```python
from build123d import *

# Parameters (mm, degrees)
F0_W      = 42
F0_H      = 17
F1_DEPTH  = 7
F4_DEPTH  = 25
F5_W      = 42
F5_H      = 5.6745335534
F6_DEPTH  = 10
F7_R      = 1.675
F8_DEPTH  = 25
F9_DEPTH  = 25
F10_W     = 5.7
F10_H     = 7
F11_DEPTH = 5
F12_DEPTH = 2


with BuildPart() as f1:
    # F0 (on Top) → F1 (new body)
    with BuildSketch(Plane.XY):
        with Locations((21, 8.5)):
            Rectangle(F0_W, F0_H)
    extrude(amount=F1_DEPTH)

    # F3 (on face) → F4 (cut)
    with BuildSketch(Plane(origin=(0, 17, 0), x_dir=(-1, 0, 0), z_dir=(0, 1, 0))):
        with BuildLine():
            ThreePointArc((-38.175, 3.5), (-36.5, 1.825), (-34.825, 3.5))
            ThreePointArc((-34.825, 3.5), (-36.5, 5.175), (-38.175, 3.5))
        make_face()
    extrude(amount=-F4_DEPTH, mode=Mode.SUBTRACT)

    # F5 (on face) → F6 (join)
    with BuildSketch(Plane.XY.offset(7)):
        with Locations((21, 14.1627332233)):
            Rectangle(F5_W, F5_H)
    extrude(amount=F6_DEPTH)

    # F7 (on face) → F8 (cut)
    with BuildSketch(Plane(origin=(0, 17, 0), x_dir=(-1, 0, 0), z_dir=(0, 1, 0))):
        with Locations((-36.5, 12.325)):
            Circle(F7_R)
        with Locations((-5.5, 12.325)):
            Circle(F7_R)
    extrude(amount=-F8_DEPTH, mode=Mode.SUBTRACT)

    # F2 (on face) → F9 (cut)
    with BuildSketch(Plane.XY.offset(7)):
        with BuildLine():
            ThreePointArc((23.0754310162, 5.6), (23.0938540508, 5.8496983645), (23.1, 6.1))
            ThreePointArc((23.1, 6.1), (23.0938540508, 6.3503016355), (23.0754310162, 6.6))
            ThreePointArc((23.0754310162, 6.6), (12.9, 6.1), (23.0754310162, 5.6))
        make_face()
        with BuildLine():
            Line((42, 6.1), (23.1, 6.1))
            ThreePointArc((23.1, 6.1), (23.0938540508, 5.8496983645), (23.0754310162, 5.6))
            Line((23.0754310162, 5.6), (42, 5.6))
            Line((42, 5.6), (42, 6.1))
        make_face()
        with BuildLine():
            ThreePointArc((23.0754310162, 6.6), (23.0938540508, 6.3503016355), (23.1, 6.1))
            Line((23.1, 6.1), (42, 6.1))
            Line((42, 6.1), (42, 6.6))
            Line((42, 6.6), (23.0754310162, 6.6))
        make_face()
    extrude(amount=-F9_DEPTH, mode=Mode.SUBTRACT)

    # F10 (on face) → F11 (join)
    with BuildSketch(Plane(origin=(0, 0, 0), x_dir=(0, -1, 0), z_dir=(-1, 0, 0))):
        with Locations((-11.35, 3.5)):
            Rectangle(F10_W, F10_H)
    extrude(amount=F11_DEPTH)

    # F12 (add): a face of the model
    f12_faces = [f1.faces().sort_by_distance(p)[0] for p in [
        (20.5209474116, 0, 3.5),
    ]]
    extrude(f12_faces, amount=F12_DEPTH)


solid = f1.part
```
For this review, take the finished solid that the model builds, in its own axes (mm). A direction names the side the tool comes from. Round coordinates to 2 decimals unless told otherwise and drop trailing zeros. Loops run counter-clockwise (first coordinate to the right, second up) from the corner with the lowest first, then second, coordinate; pieces in that order, holes last.
(1) Clearance check with flat-ended pins moving along their axes: P1, Ø1.7, axis at y = 14, z = 12.5, coming from the -X side; P2, Ø1, axis at x = 30, y = 3.5, coming from the +Z side; P3, Ø4, axis at x = -3.5, z = 4, coming from the -Y side. State where each tip first meets the part, or that it passes through.
Returned:
P1: stops at x = 0
P2: stops at z = 7
P3: stops at y = 8.5
(2) Mouldability with a two-part tool opening along Y and no side actions: class faces 4 (the flat face through (32, 5.6, 4)), 5 (the flat face through (21, 17, 8)), 6 (the flat face through (23, 8, 0)), 7 (the flat face through (33, 6.6, 4)) as released by +Y, released by -Y, zero draft, split by the parting line, or undercut.
Returned:
face 4: undercut
face 5: released by +Y
face 6: zero draft
face 7: undercut
(3) We need section B-B (x = 18). Give the boundary of the cut face in (y, z), plus the area to 3 significant figures.
Returned:
outline: (-2, 0) - (1, 0) - (1, 7) - (-2, 7) - close; (11.2, 0) - (17, 0) - (17, 17) - (11.33, 17) - (11.33, 7) - (11.2, 7) - close
area: 118 mm2
(4) We need section D-D (x = 36.5). Give the boundary of the cut face in (y, z) (3 decimals), plus the area to 3 significant figures.
Returned:
outline: (-2, 0) - (5.6, 0) - (5.6, 1.825) - (-2, 1.825) - close; (-2, 5.175) - (5.6, 5.175) - (5.6, 7) - (-2, 7) - close; (6.6, 0) - (17, 0) - (17, 1.825) - (6.6, 1.825) - close; (6.6, 5.175) - (17, 5.175) - (17, 10.65) - (11.325, 10.65) - (11.325, 7) - (6.6, 7) - close; (11.325, 14) - (17, 14) - (17, 17) - (11.325, 17) - close
area: 103 mm2
(5) We need section C-C (y = 9). Give the boundary of the cut face in (x, z) (3 decimals), plus the area to 3 significant figures.
Returned:
outline: (-5, 0) - (13.805, 0) - (13.805, 7) - (-5, 7) - close; (22.195, 0) - (42, 0) - (42, 7) - (22.195, 7) - close; hole circle Ø3.35 at (36.5, 3.5)
area: 261 mm2
(6) Wall thickness on line 1 along Z through (x, y) = (36.5, 14) (3 decimals); line 2 along Z through (x, y) = (5.5, 15.6); line 3 along Y through (x, z) = (18, 1.25): over which ranges is each line inside the solid? List them lowest first.
Returned:
line 1: z = 0 to 1.825, 5.175 to 10.65, 14 to 17
line 2: z = 0 to 10.65, 14 to 17
line 3: y = -2 to 1, 11.2 to 17
(7) We need section A-A (z = 3.5). Give the boundary of the cut face in (x, y) (3 decimals), plus the area to 3 significant figures.
Returned:
outline: (-5, 8.5) - (0, 8.5) - (0, -2) - (34.825, -2) - (34.825, 5.6) - (23.075, 5.6) arc R5.1 cw (long way) to (23.075, 6.6) - (34.825, 6.6) - (34.825, 17) - (0, 17) - (0, 14.2) - (-5, 14.2) - close; (38.175, -2) - (42, -2) - (42, 5.6) - (38.175, 5.6) - close; (38.175, 6.6) - (42, 6.6) - (42, 17) - (38.175, 17) - close
area: 666 mm2
(8) Tool access review of faces 1 (the flat face through (-2, 14.2, 3)), 2 (the flat face through (21, 11.325, 12)), 3 (the flat face through (-2, 8.5, 3)): name each direction out of +Z, -Z, +X, -X, +Y, -Y from which nothing blocks a thin tool from reaching the whole face with its end or side.
Returned:
face 1: +Z, -Z, -X, +Y
face 2: +Z, +X, -X, -Y
face 3: +Z, -Z, -X, -Y
